from build123d import *

# Parameters (mm, degrees)
BOSS_EXTRUDE1_DEPTH = 3
SKETCH2_R           = 2.5
CUT_EXTRUDE1_DEPTH  = 20
SKETCH3_W           = 5
SKETCH3_H           = 5
CUT_EXTRUDE2_DEPTH  = 10
SKETCH4_R           = 4.1
CUT_EXTRUDE3_DEPTH  = 10
SKETCH5_R           = 3.2
CUT_EXTRUDE4_DEPTH  = 10


with BuildPart() as part:
    # Sketch1 → Boss-Extrude1 (new body)
    with BuildSketch(Plane(origin=(0, 0, 0), x_dir=(1, 0, 0), z_dir=(0, 1, 0))):
        with BuildLine():
            Line((-19.801702617, 0), (17.198297383, 0))
            Line((17.198297383, 0), (17.198297383, 37))
            ThreePointArc((17.198297383, 37), (30.611248287, 20.881727984), (28.698297383, 0))
            Line((28.698297383, 0), (28.698297383, -30))
            Line((28.698297383, -30), (-31.301702617, -30))
            Line((-31.301702617, -30), (-31.301702617, 0))
            ThreePointArc((-31.301702617, 0), (-33.214653521, 20.881727984), (-19.801702617, 37))
            Line((-19.801702617, 37), (-19.801702617, 0))
        make_face()
    extrude(amount=BOSS_EXTRUDE1_DEPTH)

    # Sketch2 → Cut-Extrude1 (cut)
    with BuildSketch(Plane(origin=(0, 3, 0), x_dir=(1, 0, 0), z_dir=(0, 1, 0))):
        with Locations(Location((-1.301702617, -25, 0), (0, 0, 270))):
            Circle(SKETCH2_R)
    extrude(amount=-CUT_EXTRUDE1_DEPTH, mode=Mode.SUBTRACT)

    # Sketch3 → Cut-Extrude2 (cut)
    with BuildSketch(Plane.XZ):
        with Locations((13.798297383, 9.5)):
            Rectangle(SKETCH3_W, SKETCH3_H)
        with Locations((-16.401702617, 9.5)):
            Rectangle(SKETCH3_W, SKETCH3_H)
    extrude(amount=-CUT_EXTRUDE2_DEPTH, mode=Mode.SUBTRACT)

    # Sketch4 → Cut-Extrude3 (cut)
    with BuildSketch(Plane.XZ):
        with Locations(Location((13.798297383, 9.5, 0), (0, 0, 270))):
            Circle(SKETCH4_R)
        with Locations(Location((-16.401702617, 9.5, 0), (0, 0, 90))):
            Circle(SKETCH4_R)
    extrude(amount=-CUT_EXTRUDE3_DEPTH, mode=Mode.SUBTRACT)

    # Sketch5 → Cut-Extrude4 (cut)
    with BuildSketch(Plane(origin=(0, 3, 0), x_dir=(1, 0, 0), z_dir=(0, 1, 0))):
        with Locations(Location((-5.901702617, -9.5, 0), (0, 0, 270))):
            Circle(SKETCH5_R)
        with Locations(Location((3.298297383, -9.5, 0), (0, 0, 270))):
            Circle(SKETCH5_R)
    extrude(amount=-CUT_EXTRUDE4_DEPTH, mode=Mode.SUBTRACT)


solid = part.part
The listing builds one solid part. Answer for the finished solid, in the listing's coordinates (mm). A direction names the side the tool comes from. Coordinates: 2 decimals unless noted, no trailing zeros. Write each loop counter-clockwise with the first axis right and the second up, starting at its lowest first coordinate (ties: lowest second). Pieces come first, ordered by that corner, then holes. Notation, with made-up numbers: M 40.5,-29 L 59.5,-29 A18 cw 59.5,1 Z; hole C 35,17 d10. An arc over 180 degrees is marked long. Use one line per item in the form item = value.
Item 1: Find the intervals of material crossed by probe 1 along X at (y, z) = (2.2, 9.5); probe 2 along Z at (x, y) = (0.5, 2.3); probe 3 along Z at (x, y) = (13.5, 1.35), in increasing order.
Model answer:
probe_1 = -31.3 to -20.5, -12.3 to -9.1, -2.7 to 0.1, 6.5 to 9.7, 17.9 to 28.7
probe_2 = 0 to 7.95, 11.05 to 23.27, 26.73 to 30
probe_3 = 0 to 5.41, 13.59 to 30
Item 2: Find section D-D, the plane y = 1. Give the vertices of the cut face in (x, z), plus the area to 3 significant figures.
Model answer:
outline = M -31.3,0 A27.4 ccw -19.8,-37 L -19.8,0 L 17.2,0 L 17.2,-37 A27.4 ccw 28.7,0 L 28.7,30 L -31.3,30 Z; hole C -16.4,9.5 d8.2; hole C -5.9,9.5 d6.4; hole C -1.3,25 d5; hole C 3.3,9.5 d6.4; hole C 13.8,9.5 d8.2
area = 2,460 mm2
Item 3: Find section C-C, the plane x = -14.5. Give the vertices of the cut face in (y, z).
Model answer:
outline = M 0,0 L 3,0 L 3,5.87 L 0,5.87 Z; M 0,13.13 L 3,13.13 L 3,30 L 0,30 Z
Item 4: Find section A-A, the plane z = 25. Give the vertices of the cut face in (x, y).
Model answer:
outline = M -31.3,0 L -3.8,0 L -3.8,3 L -31.3,3 Z; M 1.2,0 L 28.7,0 L 28.7,3 L 1.2,3 Z
Item 5: Find section B-B, the plane z = 9.5. Give the vertices of the cut face in (x, y).
Model answer:
outline = M -31.3,0 L -20.5,0 L -20.5,3 L -31.3,3 Z; M -12.3,0 L -9.1,0 L -9.1,3 L -12.3,3 Z; M -2.7,0 L 0.1,0 L 0.1,3 L -2.7,3 Z; M 6.5,0 L 9.7,0 L 9.7,3 L 6.5,3 Z; M 17.9,0 L 28.7,0 L 28.7,3 L 17.9,3 Z
Item 6: The mould has two halves that part along Z. Classify faces 4 (the face through (-2, 1, 0)), 5 (the face through (6.47, 1.52, 9.08)), 6 (the face through (-1, 1, 30)): released by +Z, released by -Z, zero draft, split by the parting line, or undercut.
Model answer:
face_4 = released by -Z
face_5 = undercut
face_6 = released by +Z
Item 7: For faces 1 (the face through (28.698, 1, 15)), 2 (the face through (-19.802, 1, -19)), 3 (the face through (-31.302, 1, 15)), determine the directions among +Z, -Z, +X, -X, +Y, -Y from which every point of the face is accessible in a straight line to the end or side of a thin tool.
Model answer:
face_1 = +Z, +X, +Y, -Y
face_2 = -Z, +Y, -Y
face_3 = +Z, -X, +Y, -Y
Item 8: Given P1, Ø0.9, axis at y = 1, z = 16, coming from the +X side; P2, Ø1, axis at y = 1, z = -29.5, coming from the -X side; P3, Ø0.9, axis at y = 2, z = 12.5, coming from the -X side, each flat-ended and moving along its own axis, determine where each tip first touches the part or whether it passes through.
Model answer:
P1 = 28.7
P2 = -29.11
P3 = -31.3
